Work out the finished part from the listing and answer in its coordinate system (mm). Coordinates: 2 decimals unless noted, no trailing zeros. Order: outer loops, then holes, each group sorted by start corner. A loop starts at its lowest first (then second) coordinate and runs counter-clockwise, first axis right, second up. Notation, with made-up numbers: (81, 89.25) -> (131, 89.25) arc R26 cw to (131, 123.25) -> close; hole circle Ø5 at (44, -31.5). An arc over 180 degrees is marked (long way). Answer as CSV lines item,"result". Start each with the question number.
Item 1: This flat-tipped pin is pushed along its axis until it touches: pin 1 Ø0.8 at (x, z) = (0, -174.5) entering from +Y. Where does it stop, or does it pass through?
Item 2: Straight lines are drawn through the part: L1, parallel to Y at x = -0.5, z = -180.5; L2, parallel to Z at x = -0.1, y = 19.5; L3, parallel to Y at x = 0.4, z = -273.5. For each, find the intervals that lie inside material, in ascending order.
Item 3: Section A-A (x = 0.3) is taken. Write down the section's boundary in (y, z), then the cut area to 3 significant figures.
Item 4: Section B-B (z = -160.5) is taken. Write down the section's boundary in (x, y).
Item 5: Section C-C (y = 185) is taken. Write down the section's boundary in (x, z).
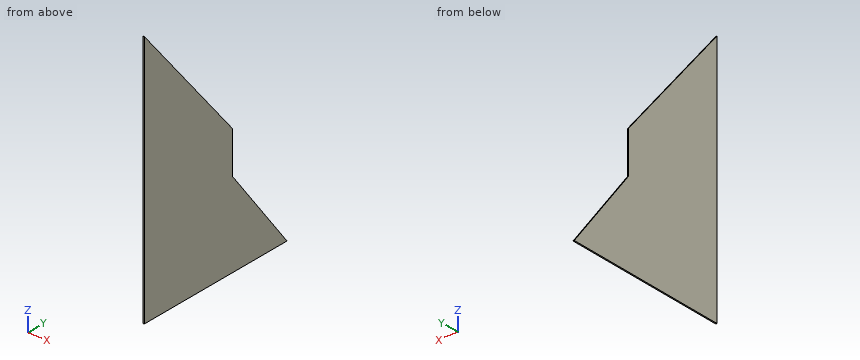
Autodesk Inventor part; units mm, degrees
ref_plane "YZ Plane" through (0, 0, 0) normal (1, 0, 0) x (0, 1, 0)
ref_plane "XZ Plane" through (0, 0, 0) normal (0, 1, 0) x (-1, 0, 0)
ref_plane "XY Plane" through (0, 0, 0) normal (0, 0, 1) x (1, 0, 0)
sketch "Boceto1" plane through (0, 0, 0) normal (1, 0, 0) x (0, 1, 0)
  line L0 (1.2642, 8.9824) -> (1.2642, -291.0176)
  line L1 (1.2642, -291.0176) -> (201.2642, -291.0176)
  line L2 (1.2642, 8.9824) -> (125.2111, -141.0176)
  line L3 (125.2111, -141.0176) -> (125.2111, -191.0176)
  line L4 (125.2111, -191.0176) -> (201.2642, -291.0176)
  point P0 (0, 0)
  dimension "d0" = 300
  dimension "d1" = 200
  dimension "d4" = 50
extrude "Extrusión1" add sketch "Boceto1" along normal mid plane 1.5
properties part number "parte lateral"
Checked values:
1,pin 1,"stops at y = 125.21"
2,L1,"y = 1.26 to 125.21"
2,L2,"z = -291.02 to -13.09"
2,L3,"y = 1.26 to 187.94"
3,outline,"(1.26, -291.02) -> (201.26, -291.02) -> (125.21, -191.02) -> (125.21, -141.02) -> (1.26, 8.98) -> close"
3,area,"31,700 mm^2"
4,outline,"(-0.75, 1.26) -> (0.75, 1.26) -> (0.75, 125.21) -> (-0.75, 125.21) -> close"
5,outline,"(-0.75, -291.02) -> (0.75, -291.02) -> (0.75, -269.63) -> (-0.75, -269.63) -> close"
